from build123d import *

# Parameters (mm, degrees)
SKETCH1_W           = 5
SKETCH1_H           = 40
BOSS_EXTRUDE1_DEPTH = 5


with BuildPart() as part:
    # Sketch1 → Boss-Extrude1 (new body)
    with BuildSketch(Plane.XY):
        Polygon((203.486718192, 206.341782002), (191.685694536, 206.341782002), (191.685694536, 161.341782002), (186.685694536, 161.341782002), (186.685694536, 206.341782002), (181.685694536, 206.341782002), (181.685694536, 201.341782002), (166.685694536, 201.341782002), (166.685694536, 206.341782002), (156.685694536, 206.341782002), (156.685694536, 201.341782002), (141.685694536, 201.341782002), (141.685694536, 206.341782002), (136.685694536, 206.341782002), (136.685694536, -243.658217998), (141.685694536, -243.658217998), (141.685694536, -238.658217998), (156.685694536, -238.658217998), (156.685694536, -243.658217998), (166.685694536, -243.658217998), (166.685694536, -238.658217998), (181.685694536, -238.658217998), (181.685694536, -243.658217998), (186.685694536, -243.658217998), (186.685694536, -198.658217998), (191.685694536, -198.658217998), (191.685694536, -243.658217998), (203.486718192, -243.658217998), align=None)
        with Locations((189.185694536, -138.658217998)):
            Rectangle(SKETCH1_W, SKETCH1_H, mode=Mode.SUBTRACT)
        with Locations((189.185694536, -58.658217998)):
            Rectangle(SKETCH1_W, SKETCH1_H, mode=Mode.SUBTRACT)
        with Locations((189.185694536, 21.341782002)):
            Rectangle(SKETCH1_W, SKETCH1_H, mode=Mode.SUBTRACT)
        with Locations((189.185694536, 101.341782002)):
            Rectangle(SKETCH1_W, SKETCH1_H, mode=Mode.SUBTRACT)
    extrude(amount=BOSS_EXTRUDE1_DEPTH)


solid = part.part
Source: CAD feature listing. Evaluate the final solid. Frame: model axes, mm. Give positions to 0.01 mm unless a question says otherwise; leave off trailing zeros. Write each loop counter-clockwise with the first axis right and the second up, starting at its lowest first coordinate (ties: lowest second). Pieces come first, ordered by that corner, then holes. Notation, with made-up numbers: M 64.5,54 L 117.5,54 A30 cw 117.5,76 Z; hole C 21.5,23 d5. An arc over 180 degrees is marked long. Return JSON: item names as keys, results as strings. Group by question number.
1) First-contact query: pin 1 Ø1.5 at (x, z) = (189.5, 3.5) entering from -Y; pin 2 Ø1.5 at (x, z) = (189, 3) entering from +Y; pin 3 Ø2.5 at (x, z) = (147, 2.5) entering from -Y; pin 4 Ø2 at (x, z) = (156, 3.5) entering from -Y. Flat tips, straight axial feed; report the tip coordinate or a pass-through.
2) Cut plane C-C, the plane x = 176. Output: boundary loops of the cut face in (y, z).
3) Ray query, L1, parallel to Y at x = 190, z = 3.25; L2, parallel to X at y = -120, z = 2.1; L3, parallel to Y at x = 175.5, z = 0.55. Return the intervals inside material, ascending.
4) Cut plane B-B, the plane z = 3.7. Give the number of separate pieces and of enclosed holes in the cut face, then the cut area to 3 significant figures.
5) Cut plane A-A, the plane y = -55. Output: boundary loops of the cut face in (x, z), then the cut area to 3 significant figures.
Data:
{
 "1": {"pin 1": "stops at y = -198.66", "pin 2": "stops at y = 161.34", "pin 3": "stops at y = -238.66", "pin 4": "stops at y = -243.66"},
 "2": {"outline": "M -238.66,0 L 201.34,0 L 201.34,5 L -238.66,5 Z"},
 "3": {"L1": "y = -198.66 to -158.66, -118.66 to -78.66, -38.66 to 1.34, 41.34 to 81.34, 121.34 to 161.34", "L2": "x = 136.69 to 186.69, 191.69 to 203.49", "L3": "y = -238.66 to 201.34"},
 "4": {"separate pieces": "1", "enclosed holes": "4", "area": "28,500 mm²"},
 "5": {"outline": "M 136.69,0 L 186.69,0 L 186.69,5 L 136.69,5 Z; M 191.69,0 L 203.49,0 L 203.49,5 L 191.69,5 Z", "area": "309 mm²"}
}
